Answer from the drawing. Dimensions are ordinates in mm from the lowest x, y and z of the part. A direction names the side the tool comes from. Give positions to 0.01 mm unless a question says otherwise; leave off trailing zeros. Order: outer loops, then holes, each group sorted by start corner. A loop starts at its lowest first (then second) coordinate and runs counter-clockwise, first axis right, second up. Notation, with made-up numbers: (30.25, 6) - (44.25, 6) arc R22 ccw to (44.25, 33) - close; hole circle Ø1 at (58, 33). An arc over 180 degrees is marked (long way). Answer in a Markdown table with one row per item. Add a question column.
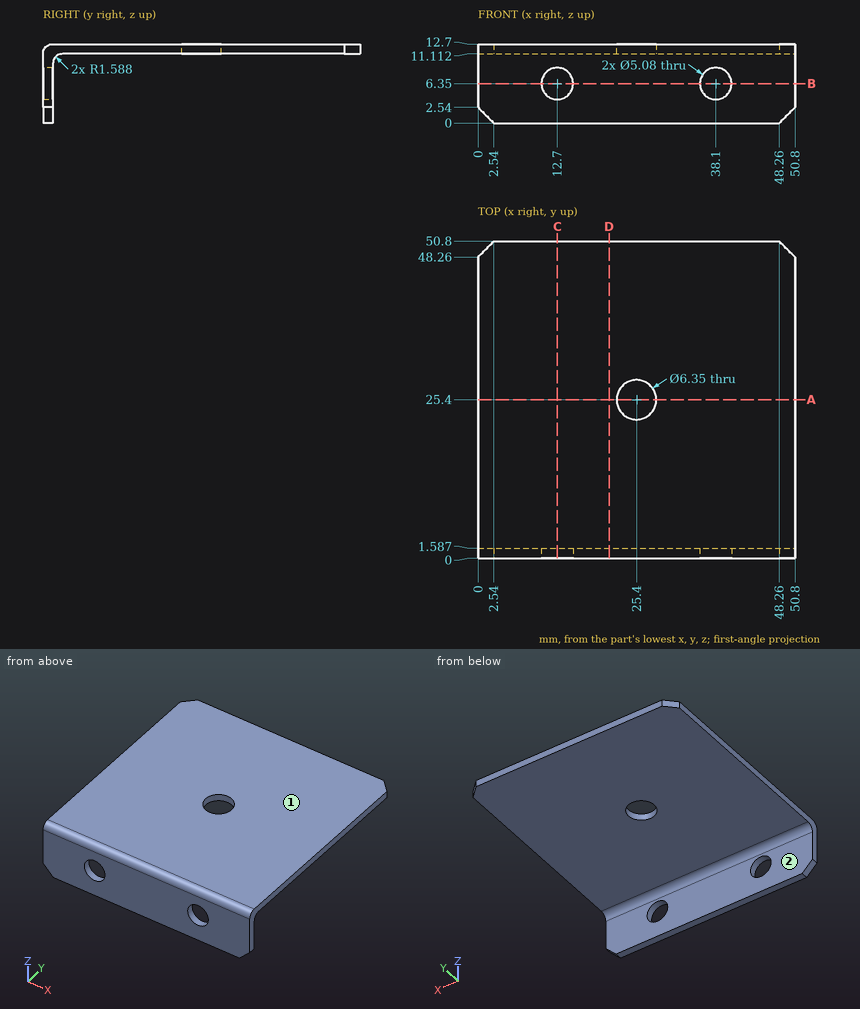
(1) Straight lines are drawn through the part: line 1 (X direction, y = 1, z = 6.35); line 2 (Z direction, x = 25.5, y = 41.5); line 3 (Y direction, x = 10, z = 6.5). For each, find the intervals that lie inside material, in ascending order.
(2) Each of these flat-tipped pins is pushed along its axis until it touches: P1, Ø1, axis at x = 35, y = 21, coming from the -Z side; P2, Ø5, axis at x = 34, z = 6.5, coming from the +Y side. Where does it stop, or does it pass through?
(3) Find section A-A, the plane y = 25.4. Write down the section's boundary in (x, z) (1 decimal).
(4) Find section B-B, the plane z = 6.35. Write down the section's boundary in (x, y).
(5) For the marked faces 1 and 2, determine the directions among +Z, -Z, +X, -X, +Y, -Y from which every point of the face is accessible in a straight line to the end or side of a thin tool.
(6) Find section D-D, the plane x = 21. Write down the section's boundary in (y, z) (1 decimal).
(7) Find section C-C, the plane x = 12.7. Write down the section's boundary in (y, z) (1 decimal).
Answer key:
| question | item | result |
|---|---|---|
| 1 | line 1 | 0 to 10.16, 15.24 to 35.56, 40.64 to 50.8 |
| 1 | line 2 | 11.11 to 12.7 |
| 1 | line 3 | 0 to 1.59 |
| 2 | P1 | z = 11.11 |
| 2 | P2 | y = 1.59 |
| 3 | outline | (0, 11.1) - (22.2, 11.1) - (22.2, 12.7) - (0, 12.7) - close; (28.6, 11.1) - (50.8, 11.1) - (50.8, 12.7) - (28.6, 12.7) - close |
| 4 | outline | (0, 0) - (10.16, 0) - (10.16, 1.59) - (0, 1.59) - close; (15.24, 0) - (35.56, 0) - (35.56, 1.59) - (15.24, 1.59) - close; (40.64, 0) - (50.8, 0) - (50.8, 1.59) - (40.64, 1.59) - close |
| 5 | face 1 | +Z, +X, -X, +Y, -Y |
| 5 | face 2 | -Z, +X, -X, +Y |
| 6 | outline | (0, 0) - (1.6, 0) - (1.6, 9.5) arc R1.6 cw to (3.2, 11.1) - (50.8, 11.1) - (50.8, 12.7) - (1.6, 12.7) arc R1.6 ccw to (0, 11.1) - close |
| 7 | outline | (0, 0) - (1.6, 0) - (1.6, 3.8) - (0, 3.8) - close; (0, 8.9) - (1.6, 8.9) - (1.6, 9.5) arc R1.6 cw to (3.2, 11.1) - (50.8, 11.1) - (50.8, 12.7) - (1.6, 12.7) arc R1.6 ccw to (0, 11.1) - close |
